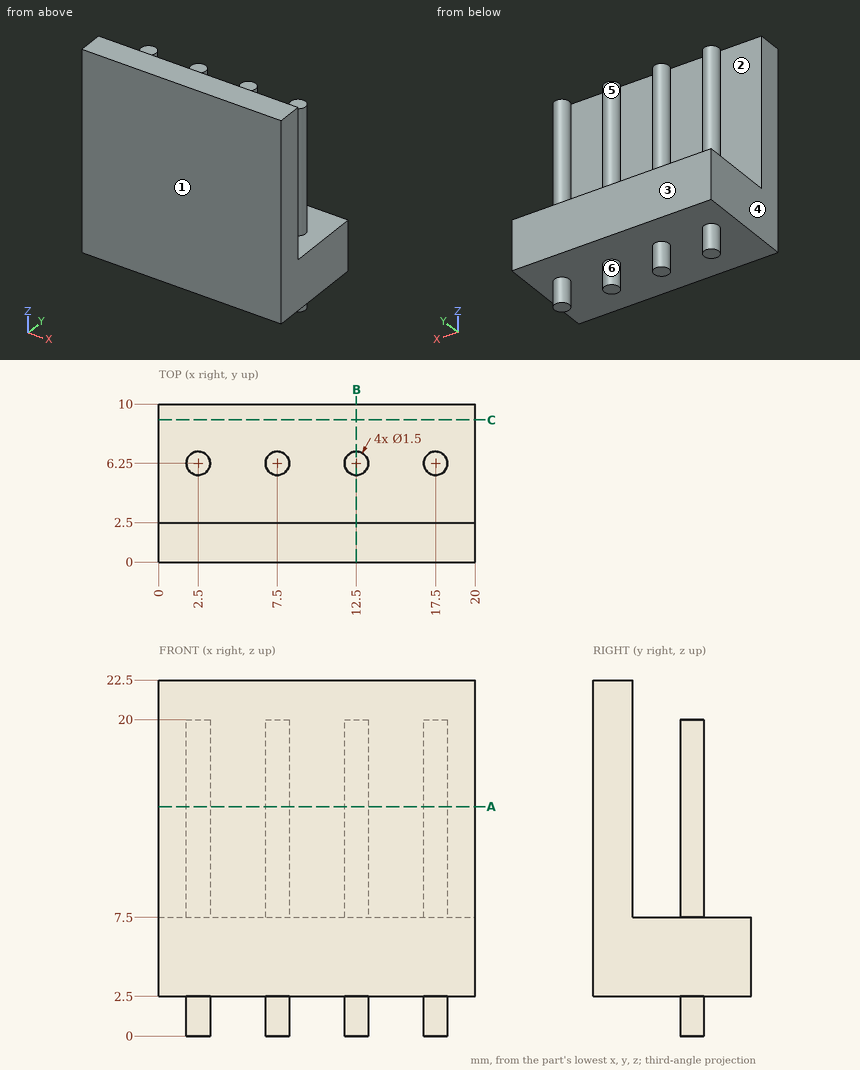
Drawing for the job (mm, zero at the part's lowest x, y, z). A direction names the side the tool comes from. Round coordinates to 2 decimals unless told otherwise and drop trailing zeros. Order: outer loops, then holes, each group sorted by start corner. A loop starts at its lowest first (then second) coordinate and runs counter-clockwise, first axis right, second up. Notation, with made-up numbers: (78, 20) -> (98, 20) arc R21 ccw to (98, 56) -> close; hole circle Ø4 at (22, 14). An arc over 180 degrees is marked (long way). Put each result on its own line as item: value.
Q1. Band-saw the part on A-A (z = 14.5). Give the cut face in (x, y).
From the geometry:
outline: (0, 0) -> (20, 0) -> (20, 2.5) -> (0, 2.5) -> close; circle Ø1.5 at (2.5, 6.25); circle Ø1.5 at (7.5, 6.25); circle Ø1.5 at (12.5, 6.25); circle Ø1.5 at (17.5, 6.25)
Q2. Wall check: line 1 (X direction, y = 6, z = 10); line 2 (Z direction, x = 1, y = 9); line 3 (Z direction, x = 17.25, y = 6.75). Give the ranges that are in metal, low to high. Write a range as [from, to].
From the geometry:
line 1: x = [1.79, 3.21], [6.79, 8.21], [11.79, 13.21], [16.79, 18.21]
line 2: z = [2.5, 7.5]
line 3: z = [0, 20]
Q3. Band-saw the part on C-C (y = 9). Give the cut face in (x, z).
From the geometry:
outline: (0, 2.5) -> (20, 2.5) -> (20, 7.5) -> (0, 7.5) -> close
Q4. Band-saw the part on B-B (x = 12.5). Give the cut face in (y, z), and give its area (3 significant figures).
From the geometry:
outline: (0, 2.5) -> (5.5, 2.5) -> (5.5, 0) -> (7, 0) -> (7, 2.5) -> (10, 2.5) -> (10, 7.5) -> (7, 7.5) -> (7, 20) -> (5.5, 20) -> (5.5, 7.5) -> (2.5, 7.5) -> (2.5, 22.5) -> (0, 22.5) -> close
area: 110 mm2
Q5. Pin check, flat tips, straight feed: pin 1 Ø12 at (x, z) = (12.5, 17.5) entering from +Y; pin 2 Ø1.6 at (x, y) = (17, 6) entering from +Z; pin 3 Ø12 at (x, z) = (15, 14) entering from -Y; pin 4 Ø1.5 at (x, y) = (8.5, 5) entering from +Z. Stop position of each tip, or through.
From the geometry:
pin 1: stops at y = 7
pin 2: stops at z = 20
pin 3: stops at y = 0
pin 4: stops at z = 7.5
Q6. Tool access for the marked faces 4, 5 and 6: list every direction of +Z, -Z, +X, -X, +Y, -Y with a clear straight run to the whole face (end or side of a thin tool).
From the geometry:
face 4: +Z, -Z, -X, +Y, -Y
face 5: +Z
face 6: -Z
Q7. Pull direction Y, two halves, no side cores. Call the marked faces 1, 2 and 3: pulls with the +Y half, pulls with the -Y half, needs draft (parallel to the pull), parting line crosses it, or undercut.
From the geometry:
face 1: pulls with the -Y half
face 2: undercut
face 3: pulls with the +Y half
